```python
from build123d import *

# Parameters (mm, degrees)
BOX015_W     = 2
BOX015_H     = 4
BOX015_DEPTH = 0.5
BOX014_W     = 2
BOX014_H     = 4
BOX014_DEPTH = 0.5
BOX004_W     = 2
BOX004_H     = 2
BOX004_DEPTH = 6
BOX001_W     = 58.5
BOX001_H     = 25
BOX001_DEPTH = 8
BOX002_W     = 61
BOX002_H     = 28
BOX002_DEPTH = 8
FILLET_R     = 1
FILLET004_R  = 0.9


with BuildPart() as obj1:
    # Box015 → Box015 (new body)
    with BuildSketch(Plane(origin=(56.25, 8, 0), x_dir=(1, 0, 0), z_dir=(0, 0, 1))):
        with Locations((1, 2)):
            Rectangle(BOX015_W, BOX015_H)
    extrude(amount=BOX015_DEPTH)


with BuildPart() as obj2:
    # Box014 → Box014 (new body)
    with BuildSketch(Plane(origin=(-5.25, 8, 0), x_dir=(1, 0, 0), z_dir=(0, 0, 1))):
        with Locations((1, 2)):
            Rectangle(BOX014_W, BOX014_H)
    extrude(amount=BOX014_DEPTH)


with BuildPart() as obj3:
    # Box004 → Box004 (new body)
    with BuildSketch(Plane(origin=(0, -4.25, -2), x_dir=(1, 0, 0), z_dir=(0, 0, 1))):
        with Locations((1, 1)):
            Rectangle(BOX004_W, BOX004_H)
    extrude(amount=BOX004_DEPTH)


with BuildPart() as obj4:
    # Sphere → Sphere (revolve)
    with BuildSketch(Plane(origin=(10, -2, 2), x_dir=(1, 0, 0), z_dir=(0, -1, 0))):
        with BuildLine():
            ThreePointArc((0, -1), (1, 0), (0, 1))
            Line((0, 1), (0, -1))
        make_face()
    revolve(axis=Axis((10, -2, 2), (0, 0, 1)))


with BuildPart() as obj5:
    # Link006 base: copy of obj4
    add(obj4.part)


with BuildPart() as obj5_1:
    # Link006 placement: moved
    add(obj5.part.moved(Location((32, 24, -0.5))))


with BuildPart() as obj5_2:
    # Link008 placement: moved
    add(obj5_1.part.moved(Location((0, 1.500002, 1))))


with BuildPart() as obj6:
    # Link005 base: copy of obj4
    add(obj4.part)


with BuildPart() as obj6_1:
    # Link005 placement: moved
    add(obj6.part.moved(Location((0, 24, -0.5))))


with BuildPart() as obj6_2:
    # Link007 placement: moved
    add(obj6_1.part.moved(Location((0, 1.5, 0.999999))))


with BuildPart() as obj7:
    # Link004 base: copy of obj4
    add(obj4.part)


with BuildPart() as obj7_1:
    # Link004 placement: moved
    add(obj7.part.moved(Location((0, -1.500001, 0.5))))


with BuildPart() as obj8:
    # Link002 base: copy of obj4
    add(obj4.part)


with BuildPart() as obj8_1:
    # Link002 placement: moved
    add(obj8.part.moved(Location((32, 0, -0.5))))


with BuildPart() as obj8_2:
    # Link003 placement: moved
    add(obj8_1.part.moved(Location((0, -1.5, 1))))


with BuildPart() as base:
    # Box001 → Box001 (new body)
    with BuildSketch(Plane(origin=(-2.75, -2.5, -2), x_dir=(1, 0, 0), z_dir=(0, 0, 1))):
        with Locations((29.25, 12.5)):
            Rectangle(BOX001_W, BOX001_H)
    extrude(amount=BOX001_DEPTH)


with BuildPart() as cut014:
    # Box002 → Box002 (new body)
    with BuildSketch(Plane(origin=(-4, -4, 0), x_dir=(1, 0, 0), z_dir=(0, 0, 1))):
        with Locations((30.5, 14)):
            Rectangle(BOX002_W, BOX002_H)
    extrude(amount=BOX002_DEPTH)

    # Cut001: cut Base
    add(base.part, mode=Mode.SUBTRACT)

    # Cut002: cut obj8
    add(obj8_2.part, mode=Mode.SUBTRACT)

    # Cut003: cut obj7
    add(obj7_1.part, mode=Mode.SUBTRACT)

    # Cut004: cut obj6
    add(obj6_2.part, mode=Mode.SUBTRACT)

    # Cut005: cut obj5
    add(obj5_2.part, mode=Mode.SUBTRACT)

    # Cut007: cut obj3
    add(obj3.part, mode=Mode.SUBTRACT)

    # Fillet
    fillet_edges = [cut014.edges().sort_by_distance(p)[0] for p in [
        (-4, 10, 8),
        (26.5, -4, 8),
        (26.5, 24, 8),
        (57, 10, 8),
    ]]
    fillet(fillet_edges, radius=FILLET_R)

    # Fillet004
    fillet004_edges = [cut014.edges().sort_by_distance(p)[0] for p in [
        (-4, -4, 3.5),
        (-4, 24, 3.5),
        (57, -4, 3.5),
        (57, 24, 3.5),
    ]]
    fillet(fillet004_edges, radius=FILLET004_R)

    # Cut: cut obj2
    add(obj2.part, mode=Mode.SUBTRACT)

    # Cut012: cut obj1
    add(obj1.part, mode=Mode.SUBTRACT)


solid = cut014.part
```
Input: part model. Units: mm. Frame: model coordinates. A direction names the side the tool comes from. Round coordinates to 2 decimals unless told otherwise and drop trailing zeros. Loops run counter-clockwise (first coordinate to the right, second up) from the corner with the lowest first, then second, coordinate; pieces in that order, holes last. Notation, with made-up numbers: (-35.75, 10.5) -> (4.25, 10.5) arc R32 ccw to (4.25, 41.5) -> close; hole circle Ø2 at (29.25, -32). An arc over 180 degrees is marked (long way). Write each question's results on one line, items separated by ' | '.
1. Set-up query: faces 1 (the face through (1, -3, 4)), 2 (the face through (26, 22.5, 3)), 3 (the face through (57, 10, 3)). Return all of +Z, -Z, +X, -X, +Y, -Y with unobstructed straight access to the full face (end or side cutting, diameter ignored); none if empty.
Geometry results:
face 1: -Z, -Y | face 2: -Z | face 3: +Z, -Z, +X, +Y, -Y
2. Ray query, line 1 (X direction, y = 8.5, z = 2.75); line 2 (Y direction, x = 29, z = 4.5); line 3 (Z direction, x = 49, y = 20.25). Return the intervals inside material, ascending. Write a range as from..to.
Geometry results:
line 1: -4..-2.75, 55.75..57 | line 2: -4..-2.5, 22.5..24 | line 3: 6..8
3. Section A-A (z = 5.25). Return loops of the section in (x, y), and give its area (3 significant figures).
Geometry results:
outline: (-4, -3.1) arc R0.9 ccw to (-3.1, -4) -> (56.1, -4) arc R0.9 ccw to (57, -3.1) -> (57, 23.1) arc R0.9 ccw to (56.1, 24) -> (-3.1, 24) arc R0.9 ccw to (-4, 23.1) -> close; hole (-2.75, -2.5) -> (55.75, -2.5) -> (55.75, 22.5) -> (-2.75, 22.5) -> close | area: 245 mm2
4. Section B-B (x = 1). Return loops of the section in (y, z), and give its area (3 significant figures).
Geometry results:
outline: (-4, 4) -> (-2.5, 4) -> (-2.5, 6) -> (22.5, 6) -> (22.5, 0) -> (24, 0) -> (24, 7) arc R1 ccw to (23, 8) -> (-3, 8) arc R1 ccw to (-4, 7) -> close | area: 67.6 mm2
5. First-contact query: P1, Ø1, axis at x = 42.5, y = 12, coming from the -Z side; P2, Ø1.2, axis at y = -3.5, z = 1.5, coming from the -X side; P3, Ø2, axis at x = 8, z = 6, coming from the -Y side; P4, Ø3.5, axis at x = 32.5, z = 4, coming from the +Y side. Flat tips, straight axial feed; report the tip coordinate or a pass-through.
Geometry results:
P1: z = 6 | P2: x = -4 | P3: y = -4 | P4: y = 24
6. Mould query, pull axis Y, two halves, no side actions, for faces 4 (the face through (26, -4, 3)), 5 (the face through (-2.75, 10, 3)), 6 (the face through (26, -2.5, 3)), 7 (the face through (2, -3, 2)). Classes: +Y half, -Y half, draft (parallel to the pull), parting line (faces both ways), or undercut.
Geometry results:
face 4: -Y half | face 5: undercut | face 6: undercut | face 7: draft
7. Section C-C (y = 14.25). Return loops of the section in (x, z).
Geometry results:
outline: (-4, 0) -> (-2.75, 0) -> (-2.75, 6) -> (55.75, 6) -> (55.75, 0) -> (57, 0) -> (57, 7) arc R1 ccw to (56, 8) -> (-3, 8) arc R1 ccw to (-4, 7) -> close
